Answer from the drawing. Dimensions are ordinates in mm from the lowest x, y and z of the part. A direction names the side the tool comes from. Coordinates: 2 decimals unless noted, no trailing zeros. Write each loop counter-clockwise with the first axis right and the second up, starting at its lowest first coordinate (ties: lowest second). Pieces come first, ordered by that corner, then holes. Notation, with made-up numbers: (52.25, 87.25) -> (57.25, 87.25) arc R16 cw to (57.25, 94.25) -> close; hole circle Ø3 at (17.25, 58). An arc over 180 degrees is marked (long way). Return JSON: item names as keys, results as strings.
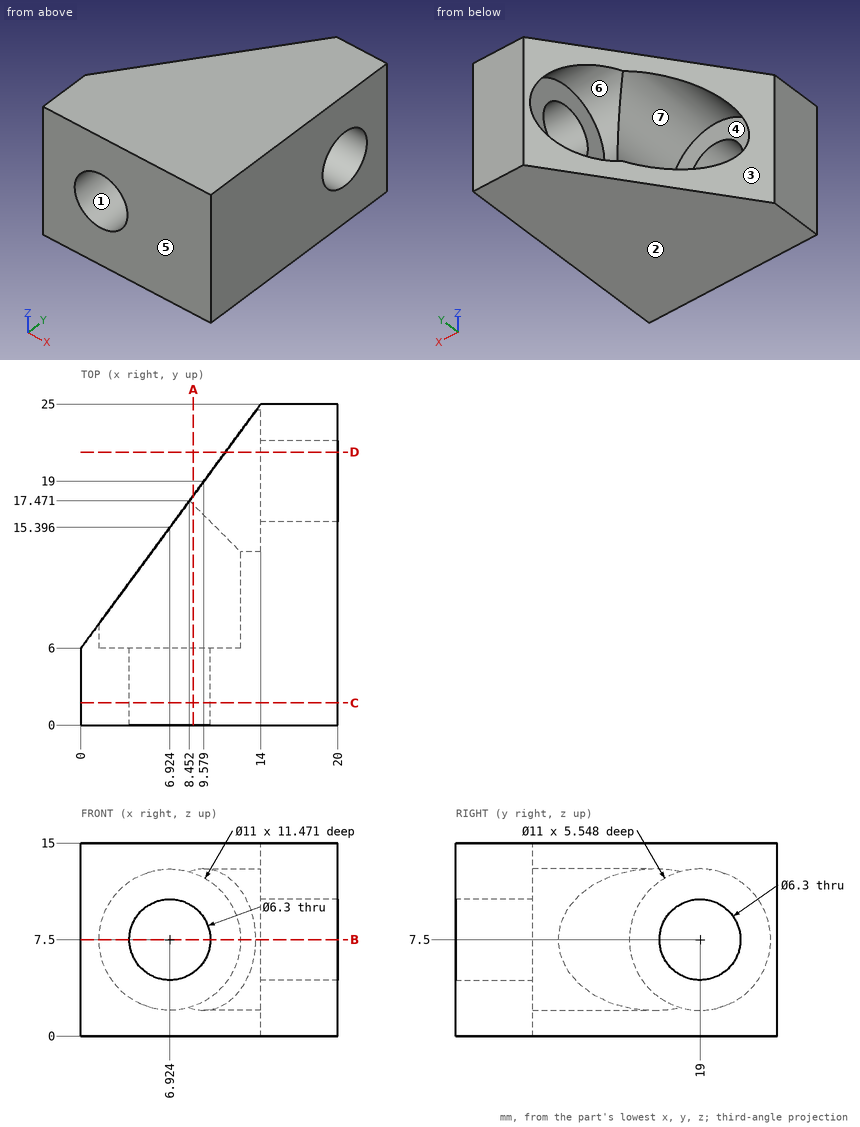
1. For a pull along X with two mould halves and no side action, classify the marked faces 1, 2, 3 and 4 as +X half, -X half, draft (parallel to the pull), parting line (faces both ways), or undercut.
Taken from the geometry:
{"face 1": "undercut", "face 2": "draft", "face 3": "-X half", "face 4": "undercut"}
2. The part is cut by section B-B (z = 7.5). Determine the outline of the cut face in (x, y), then the cut area to 3 significant figures.
Taken from the geometry:
{"outline": "(0, 0) -> (3.77, 0) -> (3.77, 6) -> (1.42, 6) -> (1.42, 7.93) -> (0, 6) -> close; (10.07, 0) -> (20, 0) -> (20, 15.85) -> (14, 15.85) -> (14, 13.5) -> (12.42, 13.5) -> (12.42, 6) -> (10.07, 6) -> close; (13.63, 24.5) -> (14, 24.5) -> (14, 22.15) -> (20, 22.15) -> (20, 25) -> (14, 25) -> close", "area": "172 mm2"}
3. Flat-ended cylindrical pins translate along their axes: pin 1 Ø5 at (y, z) = (13.5, 12.5) entering from -X (1 decimal); pin 2 Ø8 at (y, z) = (14, 11.5) entering from -X; pin 3 Ø3 at (x, z) = (10.5, 13) entering from +Y (1 decimal); pin 4 Ø2 at (x, z) = (5, 7.5) entering from +Y. Find the tip coordinate at first contact, or state that the pin passes through.
Taken from the geometry:
{"pin 1": "stops at x = 3.7", "pin 2": "stops at x = 2.95", "pin 3": "stops at y = 22.3", "pin 4": "passes through"}
4. A tool of negligible diameter and unlimited length cuts with its end or side. For the marked faces 5, 6 and 7, from which of +Z, -Z, +X, -X, +Y, -Y can it reach the whole face along a straight path? Write none if from no direction.
Taken from the geometry:
{"face 5": "+Z, -Z, +X, -X, -Y", "face 6": "-X", "face 7": "+Y"}
5. The part is cut by section A-A (x = 8.75). Determine the outline of the cut face in (y, z) (1 decimal), then the cut area to 3 significant figures.
Taken from the geometry:
{"outline": "(0, 0) -> (17.9, 0) -> (17.9, 2.1) arc R5.5 cw to (17.2, 2.3) -> (6, 2.3) -> (6, 4.9) -> (0, 4.9) -> close; (0, 10.1) -> (6, 10.1) -> (6, 12.7) -> (17.2, 12.7) arc R5.5 cw to (17.9, 12.9) -> (17.9, 15) -> (0, 15) -> close", "area": "114 mm2"}
6. Consider L1, parallel to Z at x = 16.6, y = 19; L2, parallel to X at y = 4.8, z = 7.5; L3, parallel to Y at x = 16.4, z = 7.5. Determine where each line is inside the solid, lowest interval first.
Taken from the geometry:
{"L1": "z = 0 to 4.35, 10.65 to 15", "L2": "x = 0 to 3.77, 10.07 to 20", "L3": "y = 0 to 15.85, 22.15 to 25"}
7. The part is cut by section C-C (y = 1.75). Determine the outline of the cut face in (x, z), then the cut area to 3 significant figures.
Taken from the geometry:
{"outline": "(0, 0) -> (20, 0) -> (20, 15) -> (0, 15) -> close; hole circle Ø6.3 at (6.92, 7.5)", "area": "269 mm2"}
8. The part is cut by section D-D (y = 21.25). Determine the outline of the cut face in (x, z) (1 decimal).
Taken from the geometry:
{"outline": "(11.2, 0) -> (20, 0) -> (20, 5.3) -> (14, 5.3) -> (14, 2.5) -> (11.2, 2.5) -> close; (11.2, 12.5) -> (14, 12.5) -> (14, 9.7) -> (20, 9.7) -> (20, 15) -> (11.2, 15) -> close"}
